CAD build for the part. Positions are in the model's coordinates, mm. Face numbers are marked on the shaded views. Give positions to 0.01 mm unless a question says otherwise; leave off trailing zeros. Loops run counter-clockwise (first coordinate to the right, second up) from the corner with the lowest first, then second, coordinate; pieces in that order, holes last.
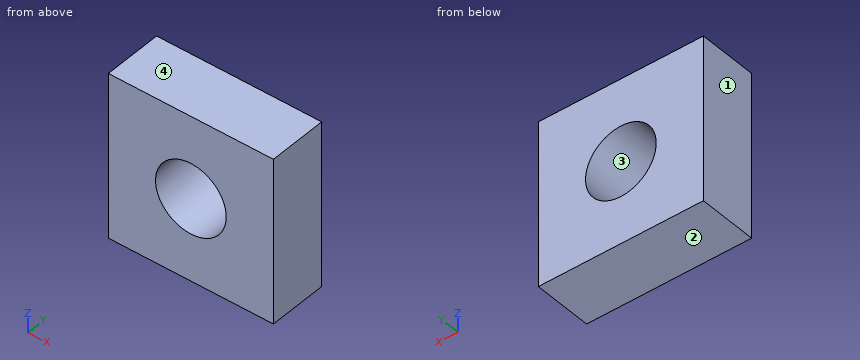
```python
from build123d import *

# Parameters (mm, degrees)
F0_W     = 70
F0_H     = 70
F1_DEPTH = 25
F2_R     = 15
F3_DEPTH = 25


with BuildPart() as f1:
    # F0 (on Front) → F1 (new body)
    with BuildSketch(Plane.XZ):
        Rectangle(F0_W, F0_H)
    extrude(amount=F1_DEPTH)

    # F2 (on Front) → F3 (cut)
    with BuildSketch(Plane.XZ):
        Circle(F2_R)
    extrude(amount=F3_DEPTH, mode=Mode.SUBTRACT)


solid = f1.part
```
1. Saw through at A-A, the plane z = 0. List the corners of the cut face in (x, y).
Responses:
outline: (-35, -25) - (-15, -25) - (-15, 0) - (-35, 0) - close; (15, -25) - (35, -25) - (35, 0) - (15, 0) - close
2. Probe line 1 along Z through (x, y) = (0, -7); line 2 along X through (y, z) = (-9, 10); line 3 along X through (y, z) = (-2.75, -13). List the from-to ranges inside material, lowest first.
Responses:
line 1: z = -35 to -15, 15 to 35
line 2: x = -35 to -11.18, 11.18 to 35
line 3: x = -35 to -7.48, 7.48 to 35
3. Saw through at B-B, the plane x = 0. List the corners of the cut face in (y, z), and give its area (3 significant figures).
Responses:
outline: (-25, -35) - (0, -35) - (0, -15) - (-25, -15) - close; (-25, 15) - (0, 15) - (0, 35) - (-25, 35) - close
area: 1,000 mm2
4. Pull direction Z, two halves, no side cores. Call the marked faces 1, 2, 3 and 4: released by +Z, released by -Z, zero draft, split by the parting line, or undercut.
Responses:
face 1: zero draft
face 2: released by -Z
face 3: undercut
face 4: released by +Z
5. Saw through at C-C, the plane y = -23.5. List the corners of the cut face in (x, z), and give its area (3 significant figures).
Responses:
outline: (-35, -35) - (35, -35) - (35, 35) - (-35, 35) - close; hole circle Ø30 at (0, 0)
area: 4,190 mm2
